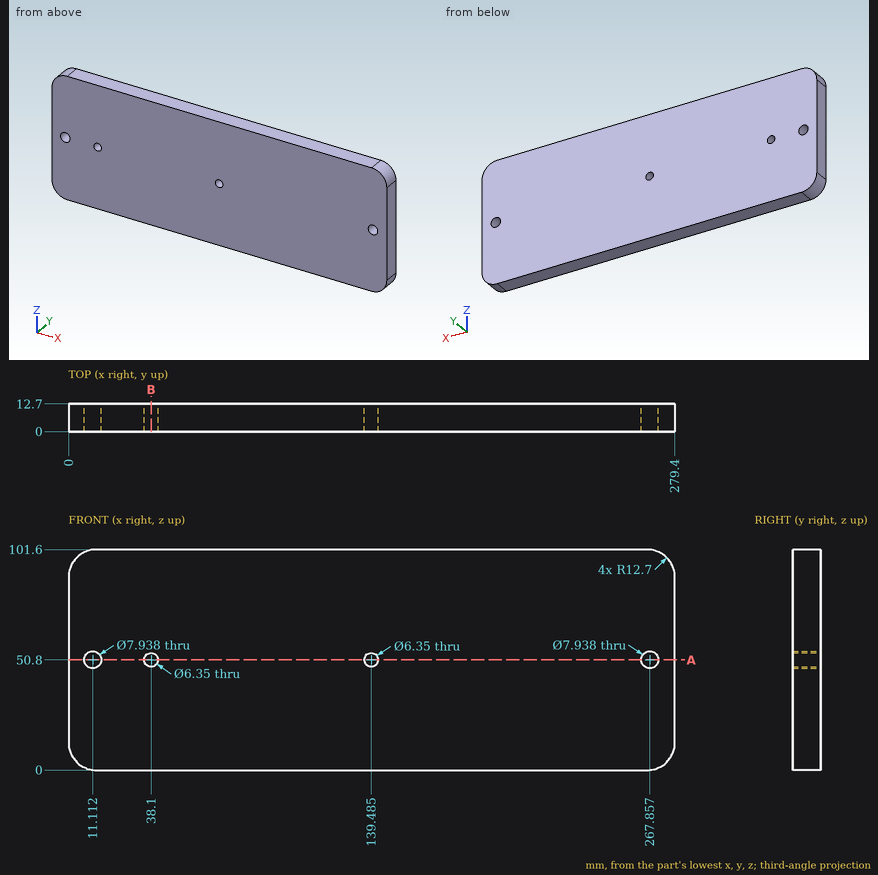
Part print with two shaded views. Sizes in mm from the minimum x, y, z corner. Give positions to 0.01 mm unless a question says otherwise; leave off trailing zeros. Order: outer loops, then holes, each group sorted by start corner. A loop starts at its lowest first (then second) coordinate and runs counter-clockwise, first axis right, second up. Notation, with made-up numbers: M 46,85.5 L 60,85.5 A27 ccw 60,119.5 Z; hole C -1.75,89 d7. An arc over 180 degrees is marked long. Write item = value, one per line.
Q1. Drill centre lines: line 1 (Z direction, x = 38.1, y = 6.75) (1 decimal); line 2 (X direction, y = 2.25, z = 52.5) (1 decimal); line 3 (X direction, y = 3.5, z = 90). Where is each one in solid material? Low to high. Write a range as [from, to].
Derived:
line_1 = [0, 47.6], [54, 101.6]
line_2 = [0, 7.5], [14.7, 35.4], [40.8, 136.8], [142.2, 264.3], [271.4, 279.4]
line_3 = [0.05, 279.35]
Q2. Cut at A-A, the plane z = 50.8. List the corners of the cut face in (x, y) (1 decimal).
Derived:
outline = M 0,0 L 7.1,0 L 7.1,12.7 L 0,12.7 Z; M 15.1,0 L 34.9,0 L 34.9,12.7 L 15.1,12.7 Z; M 41.3,0 L 136.3,0 L 136.3,12.7 L 41.3,12.7 Z; M 142.7,0 L 263.9,0 L 263.9,12.7 L 142.7,12.7 Z; M 271.8,0 L 279.4,0 L 279.4,12.7 L 271.8,12.7 Z
Q3. Cut at B-B, the plane x = 38.1. List the corners of the cut face in (y, z) (1 decimal), then the cut area to 3 significant figures.
Derived:
outline = M 0,0 L 12.7,0 L 12.7,47.6 L 0,47.6 Z; M 0,54 L 12.7,54 L 12.7,101.6 L 0,101.6 Z
area = 1,210 mm2
